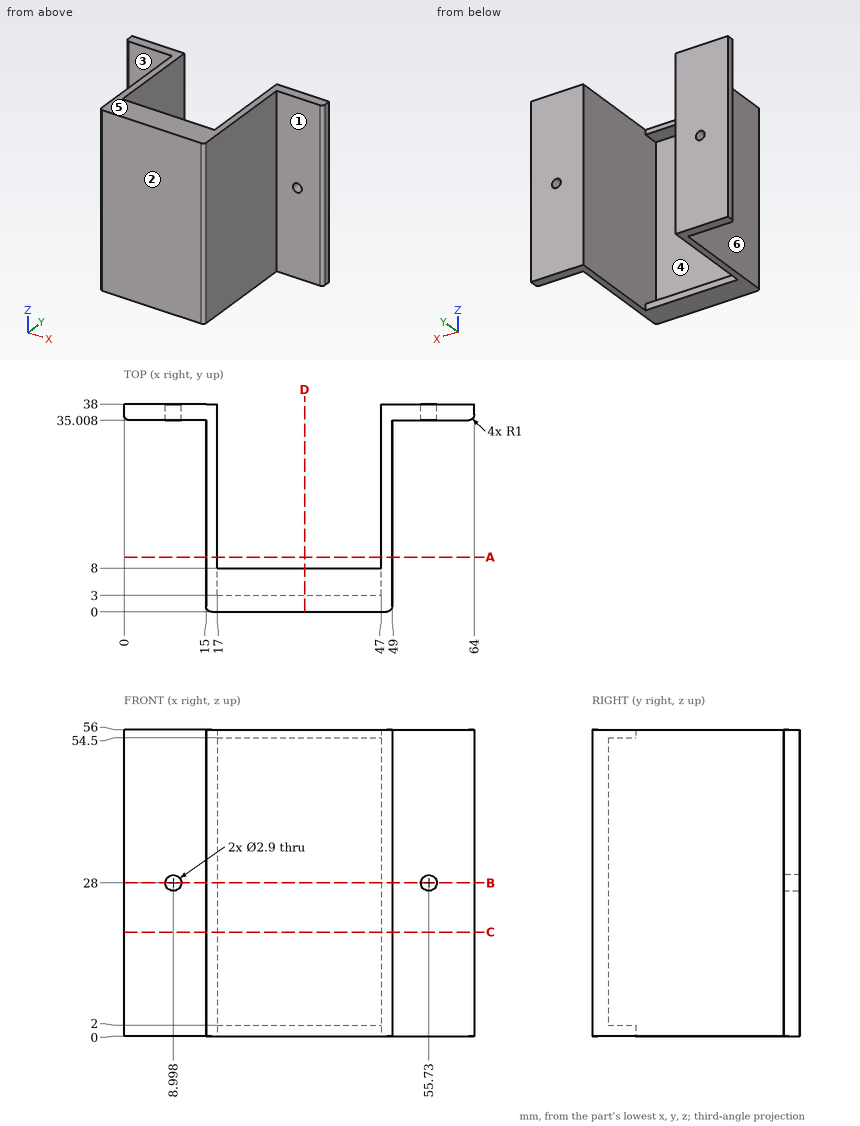
Verification items for this drawing (mm, ordinates from the low corner). A direction names the side the tool comes from. Coordinates: 2 decimals unless noted, no trailing zeros. Write each loop counter-clockwise with the first axis right and the second up, starting at its lowest first coordinate (ties: lowest second). Pieces come first, ordered by that corner, then holes. Notation, with made-up numbers: M 69.25,-20 L 102.25,-20 A15 ccw 102.25,7 Z; hole C 55.25,-11 d5. An arc over 180 degrees is marked long. Answer as CSV lines item,"result".
Q1. Set-up check for the marked faces 1, 2 and 3: record each of +Z, -Z, +X, -X, +Y, -Y from which the full face is reachable in a straight line by a thin tool's end or side.
Check result:
face 1,"+Z, -Z, +X, -Y"
face 2,"+Z, -Z, +X, -X, -Y"
face 3,"+Z, -Z, -X, -Y"
Q2. Cross-section at A-A (y = 10). Record the boundary of the cut face in (x, z), then the cut area to 3 significant figures.
Check result:
outline,"M 15,0 L 17,0 L 17,56 L 15,56 Z; M 47,0 L 49,0 L 49,56 L 47,56 Z"
area,"224 mm^2"
Q3. Material ranges on probe 1 along X at (y, z) = (36, 28); probe 2 along X at (y, z) = (19, 12.5); probe 3 along Z at (x, y) = (17.5, 6.5), recorded low to high. Write a range as from..to.
Check result:
probe 1,"0..7.55, 10.45..17, 47..54.28, 57.18..64"
probe 2,"15..17, 47..49"
probe 3,"0..2, 54.5..56"
Q4. Cross-section at D-D (x = 33). Record the boundary of the cut face in (y, z).
Check result:
outline,"M 0,0 L 8,0 L 8,2 L 3,2 L 3,54.5 L 8,54.5 L 8,56 L 0,56 Z"
Q5. Cross-section at C-C (z = 19). Record the boundary of the cut face in (x, y), then the cut area to 3 significant figures.
Check result:
outline,"M 0,36.01 A1 ccw 1,35.01 L 15,35.01 L 15,1 A1 ccw 16,0 L 48,0 A1 ccw 49,1 L 49,35.01 L 63,35.01 A1 ccw 64,36.01 L 64,38 L 47,38 L 47,3 L 17,3 L 17,38 L 0,38 Z"
area,"331 mm^2"
Q6. Mould release check, pull along X, two halves, no side actions. Record for the marked faces 4, 5 and 6: released by +X, released by -X, zero draft, split by the parting line, or undercut.
Check result:
face 4,"undercut"
face 5,"zero draft"
face 6,"released by -X"
Q7. Go/stop test with flat-tipped pins: pin 1 (1 mm diameter, centred on y = 4.5, z = 16, fed in from +X); pin 2 (10 mm diameter, centred on y = 23, z = 37, fed in from -X); pin 3 (4 mm diameter, centred on x = 11, z = 32.5, fed in from -Y). Record where each tip stops, or that it passes through.
Check result:
pin 1,"x = 49"
pin 2,"x = 15"
pin 3,"y = 35.01"
Q8. Cross-section at B-B (z = 28). Record the boundary of the cut face in (x, y).
Check result:
outline,"M 0,36.01 A1 ccw 1,35.01 L 7.55,35.01 L 7.55,38 L 0,38 Z; M 10.45,35.01 L 15,35.01 L 15,1 A1 ccw 16,0 L 48,0 A1 ccw 49,1 L 49,35.01 L 54.28,35.01 L 54.28,38 L 47,38 L 47,3 L 17,3 L 17,38 L 10.45,38 Z; M 57.18,35.01 L 63,35.01 A1 ccw 64,36.01 L 64,38 L 57.18,38 Z"
